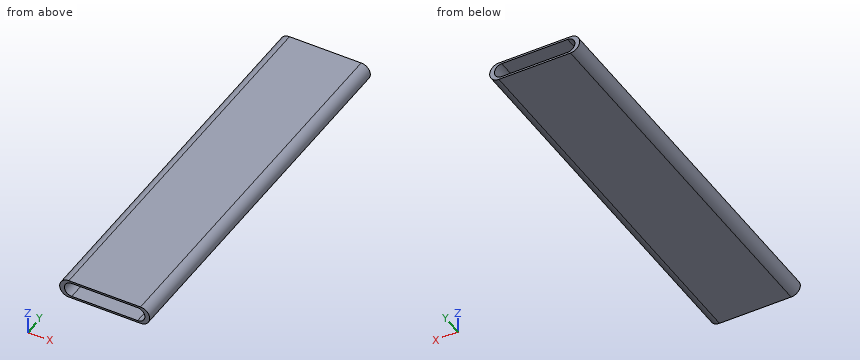
Autodesk Inventor part; units mm, degrees
ref_plane "РабПлоскость1" through (0, 210, 0) normal (0, 1, 0) x (1, 0, 0)
ref_plane "YZ Plane" through (0, 0, 0) normal (1, 0, 0) x (0, 1, 0)
ref_plane "XZ Plane" through (0, 0, 0) normal (0, 1, 0) x (-1, 0, 0)
sketch "Эскиз1" plane through (0, 0, 0) normal (0, 1, 0) x (-1, 0, 0)
  line L0 (20.5571, -2.4) -> (-16.8429, -2.4)
  line L1 (-21.6429, -7.2) -> (-21.6429, -7.2)
  line L2 (-16.8429, -12) -> (20.5571, -12)
  line L3 (25.3571, -7.2) -> (25.3571, -7.2)
  arc A0 (25.3571, -7.2) -> (20.5571, -2.4) centre (20.5571, -7.2) ccw
  arc A1 (20.5571, -12) -> (25.3571, -7.2) centre (20.5571, -7.2) ccw
  arc A2 (-16.8429, -2.4) -> (-21.6429, -7.2) centre (-16.8429, -7.2) ccw
  arc A3 (-21.6429, -7.2) -> (-16.8429, -12) centre (-16.8429, -7.2) ccw
  line L4 (19.0571, -3.4) -> (-15.3429, -3.4)
  line L5 (-19.1429, -7.2) -> (-19.1429, -7.2)
  line L6 (-15.3429, -11) -> (19.0571, -11)
  line L7 (22.8571, -7.2) -> (22.8571, -7.2)
  arc A4 (22.8571, -7.2) -> (19.0571, -3.4) centre (19.0571, -7.2) ccw
  arc A5 (19.0571, -11) -> (22.8571, -7.2) centre (19.0571, -7.2) ccw
  arc A6 (-19.1429, -7.2) -> (-15.3429, -11) centre (-15.3429, -7.2) ccw
  arc A7 (-15.3429, -3.4) -> (-19.1429, -7.2) centre (-15.3429, -7.2) ccw
  point P0 (0, 0)
  point P1 (25.3571, -2.4)
  point P2 (-21.6429, -2.4)
  dimension "d0" = 47
  dimension "d1" = 9.6
  dimension "d2" = 4.8
  dimension "d3" = 1
  dimension "d4" = 1
  dimension "d5" = 2.5
  dimension "d6" = 2.5
  dimension "d7" = 3.8
extrude "Выдавливание1" add sketch "Эскиз1" along normal blind 200
ref_plane "РабПлоскость1" through (0, 210, 0) normal (0, 1, 0) x (1, 0, 0)
properties part number "isolator"
CAD build for the part. Positions are in the model's coordinates, mm. Give positions to 0.01 mm unless a question says otherwise; leave off trailing zeros. Write each loop counter-clockwise with the first axis right and the second up, starting at its lowest first coordinate (ties: lowest second). Pieces come first, ordered by that corner, then holes. Notation, with made-up numbers: M -29.5,82.5 L 5.5,82.5 A16 cw 5.5,94.5 Z; hole C 73,53 d4. An arc over 180 degrees is marked long. Return JSON: item names as keys, results as strings. Group by question number.
(1) Band-saw the part on C-C (z = -7.2). Give the cut face in (x, y).
(2) Flat gauge pins, fed straight in: pin 1 Ø1 at (y, z) = (138.5, -10.5) entering from -X; pin 2 Ø1 at (y, z) = (170.5, -5.5) entering from +X. Where does each tip first touch, or does it go through?
(3) Band-saw the part on A-A (x = -4). Give the cut face in (y, z), and give its area (3 significant figures).
(4) Drill centre lines: L1, parallel to Z at x = 13, y = 185.5; L2, parallel to X at y = 44, z = -7.5; L3, parallel to X at y = 71, z = -5.75. Where is each one in solid material? Low to high. Write a range as [from, to].
(5) Band-saw the part on B-B (y = 122). Give the cut face in (x, z), and give its area (3 significant figures).
Entries:
{
 "1": {"outline": "M -25.36,0 L -22.86,0 L -22.86,200 L -25.36,200 Z; M 19.14,0 L 21.64,0 L 21.64,200 L 19.14,200 Z"},
 "2": {"pin 1": "stops at x = -24.46", "pin 2": "stops at x = 21.49"},
 "3": {"outline": "M 0,-12 L 200,-12 L 200,-11 L 0,-11 Z; M 0,-3.4 L 200,-3.4 L 200,-2.4 L 0,-2.4 Z", "area": "400 mm^2"},
 "4": {"L1": "z = [-12, -11], [-3.4, -2.4]", "L2": "x = [-25.35, -22.85], [19.13, 21.63]", "L3": "x = [-25.13, -22.57], [18.86, 21.42]"},
 "5": {"outline": "M -20.56,-12 L 16.84,-12 A4.8 ccw 16.84,-2.4 L -20.56,-2.4 A4.8 ccw Z; hole M -19.06,-11 L 15.34,-11 A3.8 ccw 15.34,-3.4 L -19.06,-3.4 A3.8 ccw Z", "area": "125 mm^2"}
}
